```python
from build123d import *

# Parameters (mm, degrees)
SKETCH1_W               = 14.2875
SKETCH1_H               = 9.525
SKETCH1_R               = 1.905
BOSS_EXTRUDE1_DEPTH     = 7.9375
SKETCH2_W               = 8.5725
SKETCH2_H               = 3.96875
CUT_EXTRUDE1_DEPTH      = 15.309531624
CUT_EXTRUDE2_DEPTH      = 12.692667641
CUT_EXTRUDE2_DEPTH_BACK = 12.692667641
SKETCH3_W               = 5.334
SKETCH3_H               = 1.27
SKETCH4_W               = 5.334
SKETCH4_H               = 3.96875
CUT_EXTRUDE3_DEPTH      = 2.8575
SKETCH5_W               = 5.334
SKETCH5_H               = 3.96875
CUT_EXTRUDE4_DEPTH      = 2.8575
SKETCH6_R               = 3.90525
CUT_EXTRUDE5_DEPTH      = 2.44475
FILLET2_R               = 0.9525
FILLET3_R               = 0.47625


with BuildPart() as part:
    # Sketch1 → Boss-Extrude1 (new body)
    with BuildSketch(Plane(origin=(0, 0, 0), x_dir=(1, 0, 0), z_dir=(0, 1, 0))):
        Rectangle(SKETCH1_W, SKETCH1_H)
        with Locations(Location((0, 0, 0), (0, 0, 270))):
            Circle(SKETCH1_R, mode=Mode.SUBTRACT)
    extrude(amount=BOSS_EXTRUDE1_DEPTH)

    # Sketch2 → Cut-Extrude1 (cut, through all)
    with BuildSketch(Plane.XY.offset(4.7625)):
        with Locations((0, 5.953125)):
            Rectangle(SKETCH2_W, SKETCH2_H)
    extrude(amount=-CUT_EXTRUDE1_DEPTH, mode=Mode.SUBTRACT)

    # Sketch3 → Cut-Extrude2 (cut, two sides: drawn at the far end of the back side and taken through both)
    with BuildSketch(Plane(origin=(0, 0, 0), x_dir=(0, 0, -1), z_dir=(1, 0, 0)).offset(-CUT_EXTRUDE2_DEPTH_BACK)):
        with Locations((0, 4.60375)):
            Rectangle(SKETCH3_W, SKETCH3_H)
    extrude(amount=CUT_EXTRUDE2_DEPTH + CUT_EXTRUDE2_DEPTH_BACK, mode=Mode.SUBTRACT)

    # Sketch4 → Cut-Extrude3 (cut)
    with BuildSketch(Plane(origin=(7.14375, 0, 0), x_dir=(0, 0, -1), z_dir=(1, 0, 0))):
        with Locations((0, 1.984375)):
            Rectangle(SKETCH4_W, SKETCH4_H)
    extrude(amount=-CUT_EXTRUDE3_DEPTH, mode=Mode.SUBTRACT)

    # Sketch5 → Cut-Extrude4 (cut)
    with BuildSketch(Plane.ZY.offset(7.14375)):
        with Locations((0, 1.984375)):
            Rectangle(SKETCH5_W, SKETCH5_H)
    extrude(amount=-CUT_EXTRUDE4_DEPTH, mode=Mode.SUBTRACT)

    # Sketch6 → Cut-Extrude5 (cut)
    with BuildSketch(Plane(origin=(0, 3.96875, 0), x_dir=(1, 0, 0), z_dir=(0, 1, 0))):
        with Locations(Location((0, 0, 0), (0, 0, 270))):
            Circle(SKETCH6_R)
    extrude(amount=-CUT_EXTRUDE5_DEPTH, mode=Mode.SUBTRACT)

    # Fillet2
    fillet2_edges = [part.edges().sort_by_distance(p)[0] for p in [
        (-7.14375, 3.96875, 4.7625),
        (7.14375, 3.96875, 4.7625),
        (-7.14375, 3.96875, -4.7625),
        (7.14375, 3.96875, -4.7625),
    ]]
    fillet(fillet2_edges, radius=FILLET2_R)

    # Fillet3
    fillet3_edges = [part.edges().sort_by_distance(p)[0] for p in [
        (5.23875, 7.9375, 4.7625),
        (-5.23875, 7.9375, 4.7625),
        (4.28625, 5.953125, 4.7625),
        (-4.28625, 5.953125, 4.7625),
        (6.864769209, 7.9375, 4.483519209),
        (-6.864769209, 7.9375, 4.483519209),
        (7.14375, 7.9375, 0),
        (6.864769209, 7.9375, -4.483519209),
        (5.23875, 7.9375, -4.7625),
        (4.28625, 7.9375, 0),
        (-5.23875, 7.9375, -4.7625),
        (-6.864769209, 7.9375, -4.483519209),
        (-4.28625, 7.9375, 0),
        (-7.14375, 7.9375, 0),
        (4.28625, 5.953125, -4.7625),
        (-4.28625, 5.953125, -4.7625),
    ]]
    fillet(fillet3_edges, radius=FILLET3_R)


solid = part.part
```
CAD build for the part. Positions are in the model's coordinates, mm. A direction names the side the tool comes from. Give positions to 0.01 mm unless a question says otherwise; leave off trailing zeros. Order: outer loops, then holes, each group sorted by start corner. A loop starts at its lowest first (then second) coordinate and runs counter-clockwise, first axis right, second up.
(1) Drill centre lines: L1, parallel to Z at x = 0, y = 1.15 (1 decimal); L2, parallel to X at y = 4.25, z = -3.25; L3, parallel to X at y = 0.4, z = 0 (3 decimals). Where is each one in solid material? Low to high.
(2) Tool access for faces 5 (the flat face through (6, 3, -2.667)), 6 (the flat face through (-6, 5.239, 0)), 7 (the flat face through (-6, 3, -2.667)), 8 (the cylindrical face through (6.86, 3.78, -4.49)), 9 (the flat face through (4.286, 6, 0)): list every direction of +Z, -Z, +X, -X, +Y, -Y with a clear straight run to the whole face (end or side of a thin tool).
(3) Saw through at C-C, the plane x = 0. Give the cut face in (y, z) (1 decimal), then the cut area to 3 significant figures.
(4) Saw through at A-A, the plane y = 4.25. Give the cut face in (x, z) (1 decimal).
(5) Saw through at B-B, the plane z = 0. State how many separate pieces and enclosed holes the cut face has, then the cut area to 3 significant figures.
(6) Mould opens along X. For faces 1 (the flat face through (4.286, 2, 0)), 2 (the cylindrical face through (-6.87, 3.78, -4.48)), 3 (the flat face through (1, 1.524, 2)), 4 (the flat face through (6, 7.938, 0)) say: released by +X, released by -X, zero draft, split by the parting line, or undercut.
(7) Saw through at D-D, the plane y = 0.5. Give the cut face in (x, z) (1 decimal).
(8) Flat gauge pins, fed straight in: pin 1 (3 mm diameter, centred on x = 1.5, z = 2, fed in from +Y); pin 2 (2.5 mm diameter, centred on x = 0, z = 0, fed in from -Y); pin 3 (0.9 mm diameter, centred on x = 5.5, z = 0.5, fed in from -Y); pin 4 (1.2 mm diameter, centred on y = 2, z = 1, fed in from -X). Where does each tip first touch, or does it go through?
Results found:
1. L1: z = -4.8 to -1.9, 1.9 to 4.8
1. L2: x = -7.14 to -4.29, 4.29 to 7.14
1. L3: x = -4.286 to -1.905, 1.905 to 4.286
2. face 5: +X, -Y
2. face 6: +X, -X, -Y
2. face 7: -X, -Y
2. face 8: -Z, +X, +Y, -Y
2. face 9: +Z, -Z, +Y
3. outline: (0, -4.8) - (4, -4.8) - (4, -3.9) - (1.5, -3.9) - (1.5, -1.9) - (0, -1.9) - close; (0, 1.9) - (1.5, 1.9) - (1.5, 3.9) - (4, 3.9) - (4, 4.8) - (0, 4.8) - close
3. area: 12.9 mm2
4. outline: (-7.1, -3.8) arc R1 ccw to (-6.2, -4.8) - (-4.8, -4.8) arc R0.5 ccw to (-4.3, -4.3) - (-4.3, -2.7) - (-7.1, -2.7) - close; (-7.1, 2.7) - (-4.3, 2.7) - (-4.3, 4.3) arc R0.5 ccw to (-4.8, 4.8) - (-6.2, 4.8) arc R1 ccw to (-7.1, 3.8) - close; (4.3, -4.3) arc R0.5 ccw to (4.8, -4.8) - (6.2, -4.8) arc R1 ccw to (7.1, -3.8) - (7.1, -2.7) - (4.3, -2.7) - close; (4.3, 2.7) - (7.1, 2.7) - (7.1, 3.8) arc R1 ccw to (6.2, 4.8) - (4.8, 4.8) arc R0.5 ccw to (4.3, 4.3) - close
5. separate pieces: 4
5. enclosed holes: 0
5. area: 24.3 mm2
6. face 1: released by +X
6. face 2: released by -X
6. face 3: undercut
6. face 4: zero draft
7. outline: (-7.1, -3.8) arc R1 ccw to (-6.2, -4.8) - (6.2, -4.8) arc R1 ccw to (7.1, -3.8) - (7.1, -2.7) - (4.3, -2.7) - (4.3, 2.7) - (7.1, 2.7) - (7.1, 3.8) arc R1 ccw to (6.2, 4.8) - (-6.2, 4.8) arc R1 ccw to (-7.1, 3.8) - (-7.1, 2.7) - (-4.3, 2.7) - (-4.3, -2.7) - (-7.1, -2.7) - close; hole circle Ø3.8 at (0, 0)
8. pin 1: stops at y = 3.97
8. pin 2: passes through
8. pin 3: stops at y = 5.24
8. pin 4: stops at x = -4.29
